Solid Edge part; units mm, degrees
sketch "Sketch1" plane through (0, 0, 0) normal (0, -1, 0) x (1, 0, 0)
  line L0 (-3, 0) -> (-3, -2.75)
  line L1 (-3, -2.75) -> (0, -2.75)
  line L2 (0, -2.75) -> (0, -1.5)
  line L3 (0, -1.5) -> (19.6935, -1.5)
  line L4 (19.6935, -1.5) -> (20, -1.1935)
  line L5 (20, -1.1935) -> (20, 0)
  line L6 (20, 0) -> (-3, 0)
revolve "RevolvedProtrusion1" add sketch "Sketch1" angle 360 about axis through (20, 0, 0) along (-1, 0, 0)
cosmetic_thread "Thread_1" thread depth 18.5
sketch "Sketch2" plane through (0, 0, 0) normal (0, 0, 1) x (1, 0, 0)
  line L0 (0, 1.4) -> (0.51, 1.4)
  line L1 (0.51, 1.4) -> (0.51, 1.5)
  arc A0 (0.51, 1.5) -> (0.4662, 1.5101) centre (0.51, 1.6) cw
  line L2 (0.4662, 1.5101) -> (0, 1.7375)
  line L3 (0, 1.7375) -> (0, 1.4)
revolve "RevolvedProtrusion2" add sketch "Sketch2" angle 360 about axis through (0.51, 0, 0) along (-1, 0, 0)
sketch "Sketch3" plane through (0, 0, 0) normal (0, 0, 1) x (1, 0, 0)
  line L0 (0, 1.7101) -> (0.0562, 1.7101)
  arc A0 (0.0562, 1.7101) -> (0, 1.8) centre (0.1, 1.8) cw
  line L1 (0, 1.8) -> (0, 1.7101)
revolve "RevolvedProtrusion3" add sketch "Sketch3" angle 360 about axis through (20, 0, 0) along (-1, 0, 0)
hole "Hole_1" at (-3, 0, 0) direction (1, 0, 0) diameter 2.5 depth 1.3 countersink diameter 2.91 countersink angle 120
sketch "Sketch4" plane through (0, 0, 0) normal (0, 0, 1) x (1, 0, 0)
  line L0 (-3.1, 2.45) -> (-3, 2.45)
  arc A0 (-3, 2.45) -> (-2.7, 2.75) centre (-2.7, 2.45) cw
  line L1 (-2.7, 2.75) -> (-2.7, 2.85)
  line L2 (-2.7, 2.85) -> (-3.1, 2.85)
  line L3 (-3.1, 2.85) -> (-3.1, 2.45)
revolve "RevolvedCutout1" cut sketch "Sketch4" angle 360 about axis through (-2.7, 0, 0) along (-1, 0, 0)
sketch "Sketch5" plane through (-3, 0, 0) normal (1, 0, 0) x (0, 1, 0)
  line L0 (-0.7217, 1.25) -> (-1.4434, 0)
  line L1 (-1.4434, 0) -> (-0.7217, -1.25)
  line L2 (-0.7217, -1.25) -> (0.7217, -1.25)
  line L3 (0.7217, -1.25) -> (1.4434, 0)
  line L4 (1.4434, 0) -> (0.7217, 1.25)
  line L5 (0.7217, 1.25) -> (-0.7217, 1.25)
extrude "ExtrudedCutout_1" cut sketch "Sketch5" along normal blind 1.3
sketch "Sketch6" plane through (0, 0, 0) normal (0, 0, 1) x (1, 0, 0)
  line L0 (-1.7, 0) -> (-1.7, 1.25)
  line L1 (-1.7, 1.25) -> (-0.9783, 0)
  line L2 (-0.9783, 0) -> (-1.7, 0)
revolve "RevolvedCutout2" cut sketch "Sketch6" angle 360 about axis through (-0.9783, 0, 0) along (-1, 0, 0)
properties part number "Cylinder head screw DIN 912 M3x20 07065.030.020(High)"
Verification items for the finished model (mm, model axes). A direction names the side the tool comes from. Give positions to 0.01 mm unless a question says otherwise; leave off trailing zeros. Order: outer loops, then holes, each group sorted by start corner. A loop starts at its lowest first (then second) coordinate and runs counter-clockwise, first axis right, second up. Notation, with made-up numbers: M 25.5,66.5 L 74.5,66.5 A17 cw 74.5,99.5 Z; hole C 64.25,81 d10. An arc over 180 degrees is marked long. Answer as a JSON object with one key per item and string values. Group by question number.
1) Scan lines: line 1 along X through (y, z) = (-1.7, 1.6); line 2 along Y through (x, z) = (-1.5, 0.4); line 3 along X through (y, z) = (-0.1, 0.8). Record each from-to range of solid material in increasing order. Write a range as [from, to].
2) Mould release check, pull along Y, two halves, no side actions. Record for faces 4 (the face through (0, 1, -2)), 5 (the face through (-1.331, -2.685, 0.596)), 6 (the face through (-2.356, 1.088, 0.616)): released by +Y, released by -Y, zero draft, split by the parting line, or undercut.
3) Access from +Z, -Z, +X, -X, +Y, -Y to the whole of each face (thin tool, end or side, straight path). Record for faces 1 (the face through (-2, 0, -1.25)), 2 (the face through (10.24, 0.07, 1.5)), 3 (the face through (-3, 2, 0)).
4) Cross-section at A-A (x = 12.25). Enter the section's corners in (y, z), then the cut area to 3 significant figures.
5) Depth check by flat-ended pin: pin 1 Ø2 at (x, z) = (7.5, 0.5) entering from +Y; pin 2 Ø1.5 at (x, z) = (12.5, 1) entering from -Y; pin 3 Ø2 at (x, y) = (14, -2) entering from -Z. Enter the tip coordinate at first touch or a pass-through.
Result sheet:
{
 "1": {"line 1": "x = [-3, 0]", "line 2": "y = [-2.72, -0.81], [0.81, 2.72]", "line 3": "x = [-1.44, 20]"},
 "2": {"face 4": "zero draft", "face 5": "split by the parting line", "face 6": "undercut"},
 "3": {"face 1": "-X", "face 2": "+X", "face 3": "+Z, -Z, -X, +Y, -Y"},
 "4": {"outline": "C 0,0 d3", "area": "7.07 mm2"},
 "5": {"pin 1": "stops at y = 1.5", "pin 2": "stops at y = -1.48", "pin 3": "stops at z = -1.12"}
}
